```python
from build123d import *

# Parameters (mm, degrees)
SKETCH1_W           = 70
SKETCH1_H           = 35
BOSS_EXTRUDE1_DEPTH = 30
SKETCH2_W           = 15
SKETCH2_H           = 35
CUT_EXTRUDE1_DEPTH  = 20
SKETCH3_W           = 15
SKETCH3_H           = 35
CUT_EXTRUDE2_DEPTH  = 20
SKETCH4_W           = 15
SKETCH4_H           = 10
CUT_EXTRUDE3_DEPTH  = 41
SKETCH6_W           = 20
SKETCH6_H           = 5
CUT_EXTRUDE4_DEPTH  = 41
SKETCH7_R           = 5
CUT_EXTRUDE5_DEPTH  = 36


with BuildPart() as part:
    # Sketch1 → Boss-Extrude1 (new body)
    with BuildSketch(Plane(origin=(0, 0, 0), x_dir=(1, 0, 0), z_dir=(0, 1, 0))):
        with Locations((35, 17.5)):
            Rectangle(SKETCH1_W, SKETCH1_H)
    extrude(amount=BOSS_EXTRUDE1_DEPTH)

    # Sketch2 → Cut-Extrude1 (cut)
    with BuildSketch(Plane(origin=(0, 30, 0), x_dir=(1, 0, 0), z_dir=(0, 1, 0))):
        with Locations((7.5, 17.5)):
            Rectangle(SKETCH2_W, SKETCH2_H)
    extrude(amount=-CUT_EXTRUDE1_DEPTH, mode=Mode.SUBTRACT)

    # Sketch3 → Cut-Extrude2 (cut)
    with BuildSketch(Plane(origin=(0, 30, 0), x_dir=(1, 0, 0), z_dir=(0, 1, 0))):
        with Locations((62.5, 17.5)):
            Rectangle(SKETCH3_W, SKETCH3_H)
    extrude(amount=-CUT_EXTRUDE2_DEPTH, mode=Mode.SUBTRACT)

    # Sketch4 → Cut-Extrude3 (cut)
    with BuildSketch(Plane(origin=(55, 0, 0), x_dir=(0, 0, -1), z_dir=(1, 0, 0))):
        with Locations((17.5, 25)):
            Rectangle(SKETCH4_W, SKETCH4_H)
    extrude(amount=-CUT_EXTRUDE3_DEPTH, mode=Mode.SUBTRACT)

    # Sketch6 → Cut-Extrude4 (cut)
    with BuildSketch(Plane.XY):
        with Locations((35, 27.5)):
            Rectangle(SKETCH6_W, SKETCH6_H)
    extrude(amount=-CUT_EXTRUDE4_DEPTH, mode=Mode.SUBTRACT)

    # Sketch7 → Cut-Extrude5 (cut, through all)
    with BuildSketch(Plane.XY):
        with Locations((35, 10)):
            Circle(SKETCH7_R)
    extrude(amount=-CUT_EXTRUDE5_DEPTH, mode=Mode.SUBTRACT)


solid = part.part
```
CAD build for the part. Positions are in the model's coordinates, mm. A direction names the side the tool comes from. Give positions to 0.01 mm unless a question says otherwise; leave off trailing zeros. Write each loop counter-clockwise with the first axis right and the second up, starting at its lowest first coordinate (ties: lowest second). Pieces come first, ordered by that corner, then holes. Notation, with made-up numbers: M -31,33 L 4,33 A22 cw 4,68 Z; hole C 16,-23.5 d2. An arc over 180 degrees is marked long. Return JSON: item names as keys, results as strings. Group by question number.
(1) Band-saw the part on A-A (y = 26). Give the cut face in (x, z).
(2) Band-saw the part on D-D (x = 50). Give the cut face in (y, z).
(3) Band-saw the part on C-C (z = -2). Give the cut face in (x, y).
(4) 3-axis set-ups, long thin cutter, end or side, ignore diameter. For faces 4 (the face through (62, 10, -18)), 5 (the face through (35, 24, -10)), 6 (the face through (15, 18, -17)), 7 (the face through (25, 27, -30)): which of +Z, -Z, +X, -X, +Y, -Y reach the whole face in a straight line?
(5) Flat gauge pins, fed straight in: pin 1 Ø5.5 at (y, z) = (28, -4) entering from +X; pin 2 Ø4 at (x, z) = (63, -30.5) entering from +Y; pin 3 Ø5.5 at (y, z) = (26.5, -5.5) entering from -X. Where does each tip first touch, or does it go through?
(6) Drill centre lines: L1, parallel to Y at x = 35, z = -14; L2, parallel to Z at x = 17.5, y = 25.25; L3, parallel to Y at x = 35, z = -9. Where is each one in solid material? Low to high. Write a range as [from, to].
(7) Mould opens along X. For faces 1 (the face through (20, 30, -5)), 2 (the face through (35, 25, -5)), 3 (the face through (0, 5, -17)) say: pulls with the +X half, pulls with the -X half, needs draft (parallel to the pull), parting line crosses it, or undercut.
(8) Band-saw the part on B-B (x = 35). Give the cut face in (y, z).
Entries:
{
 "1": {"outline": "M 15,-35 L 25,-35 L 25,-25 L 15,-25 Z; M 15,-10 L 25,-10 L 25,0 L 15,0 Z; M 45,-35 L 55,-35 L 55,-25 L 45,-25 Z; M 45,-10 L 55,-10 L 55,0 L 45,0 Z"},
 "2": {"outline": "M 0,-35 L 30,-35 L 30,-25 L 20,-25 L 20,-10 L 30,-10 L 30,0 L 0,0 Z"},
 "3": {"outline": "M 0,0 L 70,0 L 70,10 L 55,10 L 55,30 L 45,30 L 45,25 L 25,25 L 25,30 L 15,30 L 15,10 L 0,10 Z; hole C 35,10 d10"},
 "4": {"face 4": "+Z, -Z, +X, +Y", "face 5": "+X, -X, +Y", "face 6": "+Z, -Z, -X, +Y", "face 7": "+Z, -Z, +Y"},
 "5": {"pin 1": "stops at x = 55", "pin 2": "stops at y = 10", "pin 3": "stops at x = 15"},
 "6": {"L1": "y = [0, 5], [15, 20]", "L2": "z = [-35, -25], [-10, 0]", "L3": "y = [0, 5], [15, 25]"},
 "7": {"face 1": "needs draft", "face 2": "undercut", "face 3": "pulls with the -X half"},
 "8": {"outline": "M 0,-35 L 5,-35 L 5,0 L 0,0 Z; M 15,-35 L 25,-35 L 25,-25 L 20,-25 L 20,-10 L 25,-10 L 25,0 L 15,0 Z"}
}
